```python
from build123d import *

# Parameters (mm, degrees)
BOSS_EXTRUDE1_DEPTH     = 20
SKETCH2_W               = 5
SKETCH2_H               = 10
SKETCH2_R               = 1.6
CUT_EXTRUDE1_DEPTH      = 1
CUT_EXTRUDE1_DEPTH_BACK = 6
SKETCH2_3_R             = 2.85
SKETCH2_3_R_2           = 1.6
CUT_EXTRUDE2_DEPTH      = 1
CUT_EXTRUDE2_DEPTH_BACK = 3


with BuildPart() as part:
    # Sketch1 → Boss-Extrude1 (new body)
    with BuildSketch(Plane.YZ):
        with BuildLine():
            ThreePointArc((4.898979486, 1), (0, 5), (-4.898979486, 1))
            Line((-4.898979486, 1), (-17.5, 1))
            Line((-17.5, 1), (-17.5, 6))
            Line((-17.5, 6), (17.5, 6))
            Line((17.5, 6), (17.5, 1))
            Line((17.5, 1), (4.898979486, 1))
        make_face()
    extrude(amount=BOSS_EXTRUDE1_DEPTH)

    # Sketch2 → Cut-Extrude1 (cut, two sides)
    with BuildSketch(Plane.XY.offset(6)) as cut_extrude1_sk:
        with Locations((2.5, -12.5)):
            Rectangle(SKETCH2_W, SKETCH2_H)
        with Locations((2.5, 12.5)):
            Rectangle(SKETCH2_W, SKETCH2_H)
        with Locations((17.5, 12.5)):
            Rectangle(SKETCH2_W, SKETCH2_H)
        with Locations((17.5, -12.5)):
            Rectangle(SKETCH2_W, SKETCH2_H)
        with Locations((10, -12.5)):
            Circle(SKETCH2_R)
        with Locations((10, 12.5)):
            Circle(SKETCH2_R)
    extrude(amount=CUT_EXTRUDE1_DEPTH, mode=Mode.SUBTRACT)
    extrude(cut_extrude1_sk.sketch, amount=-CUT_EXTRUDE1_DEPTH_BACK, mode=Mode.SUBTRACT)

    # Sketch2<3> → Cut-Extrude2 (cut, two sides)
    with BuildSketch(Plane.XY.offset(6)) as cut_extrude2_sk:
        with Locations((10, -12.5)):
            Circle(SKETCH2_3_R)
        with Locations((10, -12.5)):
            Circle(SKETCH2_3_R_2, mode=Mode.SUBTRACT)
        with Locations((10, 12.5)):
            Circle(SKETCH2_3_R)
        with Locations((10, 12.5)):
            Circle(SKETCH2_3_R_2, mode=Mode.SUBTRACT)
    extrude(amount=CUT_EXTRUDE2_DEPTH, mode=Mode.SUBTRACT)
    extrude(cut_extrude2_sk.sketch, amount=-CUT_EXTRUDE2_DEPTH_BACK, mode=Mode.SUBTRACT)


solid = part.part
```
The listing builds one solid part. Answer for the finished solid, in the listing's coordinates (mm). A direction names the side the tool comes from. Give positions to 0.01 mm unless a question says otherwise; leave off trailing zeros. Order: outer loops, then holes, each group sorted by start corner. A loop starts at its lowest first (then second) coordinate and runs counter-clockwise, first axis right, second up.
Item 1: Given pin 1 Ø1.5 at (y, z) = (-12, 2.5) entering from +X; pin 2 Ø3 at (x, y) = (10.5, -12) entering from +Z; pin 3 Ø1 at (x, z) = (3.5, 3.5) entering from -Y, each flat-ended and moving along its own axis, determine where each tip first touches the part or whether it passes through.
From the geometry:
pin 1: stops at x = 15
pin 2: stops at z = 3
pin 3: stops at y = -7.5
Item 2: Which of the six approach directions +Z, -Z, +X, -X, +Y, -Y give full straight-line access (tool end or side, diameter ignored) to faces 1 (the face through (17, 7.5, 4)), 2 (the face through (17, -7.5, 4)), 3 (the face through (5, 12, 4)), 4 (the face through (2, -7.5, 4))?
From the geometry:
face 1: +Z, -Z, +X, +Y
face 2: +Z, -Z, +X, -Y
face 3: +Z, -Z, -X, +Y
face 4: +Z, -Z, -X, -Y
Item 3: Find the intervals of material crossed by probe 1 along Y at (x, z) = (10, 5.15); probe 2 along Y at (x, z) = (9.5, 3.65); probe 3 along Y at (x, z) = (9.75, 1.4), in increasing order.
From the geometry:
probe 1: y = -17.5 to -15.35, -9.65 to 9.65, 15.35 to 17.5
probe 2: y = -17.5 to -15.31, -9.69 to -3.42, 3.42 to 9.69, 15.31 to 17.5
probe 3: y = -17.5 to -14.08, -10.92 to -4.8, 4.8 to 10.92, 14.08 to 17.5
Item 4: The part is cut by section B-B, the plane z = 4.2. Give the vertices of the cut face in (x, y).
From the geometry:
outline: (0, -7.5) - (5, -7.5) - (5, -17.5) - (15, -17.5) - (15, -7.5) - (20, -7.5) - (20, -2.71) - (0, -2.71) - close; (0, 2.71) - (20, 2.71) - (20, 7.5) - (15, 7.5) - (15, 17.5) - (5, 17.5) - (5, 7.5) - (0, 7.5) - close; hole circle Ø5.7 at (10, -12.5); hole circle Ø5.7 at (10, 12.5)
Item 5: The part is cut by section A-A, the plane y = -12.5. Give the vertices of the cut face in (x, z), and give its area (3 significant figures).
From the geometry:
outline: (5, 1) - (8.4, 1) - (8.4, 3) - (7.15, 3) - (7.15, 6) - (5, 6) - close; (11.6, 1) - (15, 1) - (15, 6) - (12.85, 6) - (12.85, 3) - (11.6, 3) - close
area: 26.5 mm2
Item 6: The part is cut by section C-C, the plane x = 10. Give the vertices of the cut face in (y, z).
From the geometry:
outline: (-17.5, 1) - (-14.1, 1) - (-14.1, 3) - (-15.35, 3) - (-15.35, 6) - (-17.5, 6) - close; (-10.9, 1) - (-4.9, 1) arc R5 cw to (4.9, 1) - (10.9, 1) - (10.9, 3) - (9.65, 3) - (9.65, 6) - (-9.65, 6) - (-9.65, 3) - (-10.9, 3) - close; (14.1, 1) - (17.5, 1) - (17.5, 6) - (15.35, 6) - (15.35, 3) - (14.1, 3) - close
Item 7: The part is cut by section D-D, the plane z = 1.75. Give the vertices of the cut face in (x, y).
From the geometry:
outline: (0, -7.5) - (5, -7.5) - (5, -17.5) - (15, -17.5) - (15, -7.5) - (20, -7.5) - (20, -4.68) - (0, -4.68) - close; (0, 4.68) - (20, 4.68) - (20, 7.5) - (15, 7.5) - (15, 17.5) - (5, 17.5) - (5, 7.5) - (0, 7.5) - close; hole circle Ø3.2 at (10, -12.5); hole circle Ø3.2 at (10, 12.5)
Item 8: For a pull along Y with two mould halves and no side action, classify faces 5 (the face through (7.899, 14.426, 4.521)), 6 (the face through (10, 10, 1)), 7 (the face through (2, 7.5, 4)), 8 (the face through (11, -14, 3)) as pulls with the +Y half, pulls with the -Y half, needs draft (parallel to the pull), parting line crosses it, or undercut.
From the geometry:
face 5: undercut
face 6: needs draft
face 7: pulls with the +Y half
face 8: undercut
